Source: CAD feature listing. Evaluate the final solid. Frame: model axes, mm. Face numbers are marked on the shaded views. A direction names the side the tool comes from. Give positions to 0.01 mm unless a question says otherwise; leave off trailing zeros. Write each loop counter-clockwise with the first axis right and the second up, starting at its lowest first coordinate (ties: lowest second). Pieces come first, ordered by that corner, then holes. Notation, with made-up numbers: (32, 3) -> (80, 3) arc R29 ccw to (80, 33) -> close; hole circle Ø11 at (17.5, 64). An arc over 180 degrees is marked (long way). Write item = value, one per line.
from build123d import *

# Parameters (mm, degrees)
SKETCH1_W            = 29.21
SKETCH1_H            = 76.2
BOSS_EXTRUDE1_DEPTH  = 6.858
SKETCH3_R            = 2.032
CUT_EXTRUDE1_DEPTH   = 25.4
SKETCH17_W           = 3.81
SKETCH17_H           = 76.2
BOSS_EXTRUDE13_DEPTH = 67.818
SKETCH18_W           = 3.81
SKETCH18_H           = 20.32
BOSS_EXTRUDE14_DEPTH = 25.4
SKETCH19_W           = 29.21
SKETCH19_H           = 19.948928224
BOSS_EXTRUDE15_DEPTH = 25.4
SKETCH4_R            = 2.032
CUT_EXTRUDE5_DEPTH   = 116.113658891
SKETCH21_R           = 4
SKETCH21_R_2         = 2
CUT_EXTRUDE6_DEPTH   = 3.048
CUT_EXTRUDE7_START   = -3.048
SKETCH22_R           = 4
CUT_EXTRUDE7_DEPTH   = 3.048
SKETCH23_W           = 15.24
SKETCH23_H           = 38.1
CUT_EXTRUDE8_DEPTH   = 109.488248995
SKETCH24_W           = 24.012467883
SKETCH24_H           = 25.448429418
CUT_EXTRUDE9_DEPTH   = 10.16


with BuildPart() as part:
    # Sketch1 → Boss-Extrude1 (new body)
    with BuildSketch(Plane.XY):
        with Locations((19.297661272, -42.679075546)):
            Rectangle(SKETCH1_W, SKETCH1_H)
    extrude(amount=BOSS_EXTRUDE1_DEPTH)

    # Sketch3 → Cut-Extrude1 (cut)
    with BuildSketch(Plane.XY.offset(6.858)):
        with Locations((17.413506863, -42.679058438)):
            Circle(SKETCH3_R)
        with Locations((17.392661272, -29.979075546)):
            Circle(SKETCH3_R)
        with Locations((17.392661272, -17.279075546)):
            Circle(SKETCH3_R)
    extrude(amount=-CUT_EXTRUDE1_DEPTH, mode=Mode.SUBTRACT)

    # Sketch17 → Boss-Extrude13 (add)
    with BuildSketch(Plane(origin=(0, 0, 0), x_dir=(-1, 0, 0), z_dir=(0, 0, -1))):
        with Locations((-31.997661272, -42.679075546)):
            Rectangle(SKETCH17_W, SKETCH17_H)
    extrude(amount=BOSS_EXTRUDE13_DEPTH)

    # Sketch18 → Boss-Extrude14 (add)
    with BuildSketch(Plane.ZY.offset(-30.092661272)):
        with Locations((-65.913, -70.619075546)):
            Rectangle(SKETCH18_W, SKETCH18_H)
    extrude(amount=BOSS_EXTRUDE14_DEPTH)

    # Sketch19 → Boss-Extrude15 (add)
    with BuildSketch(Plane.ZY.offset(-30.092661272)):
        with Locations((-36.703, -70.804611434)):
            Rectangle(SKETCH19_W, SKETCH19_H)
    extrude(amount=BOSS_EXTRUDE15_DEPTH)

    # Sketch4 → Cut-Extrude5 (cut, through all)
    with BuildSketch(Plane.XY.offset(6.858)):
        with Locations((17.413506863, -68.079058438)):
            Circle(SKETCH4_R)
    extrude(amount=-CUT_EXTRUDE5_DEPTH, mode=Mode.SUBTRACT)

    # Sketch21 → Cut-Extrude6 (cut)
    with BuildSketch(Plane(origin=(0, 0, 0), x_dir=(-1, 0, 0), z_dir=(0, 0, -1))):
        with Locations((-17.413506863, -68.079058438)):
            Circle(SKETCH21_R)
        with Locations((-17.413506863, -68.079058438)):
            Circle(SKETCH21_R_2, mode=Mode.SUBTRACT)
    extrude(amount=-CUT_EXTRUDE6_DEPTH, mode=Mode.SUBTRACT)

    # Sketch22 → Cut-Extrude7 (cut)
    with BuildSketch(Plane.XY.offset(6.858).offset(CUT_EXTRUDE7_START)):
        with Locations(Location((17.413506863, -68.079058438, 0), (0, 0, 180))):
            Circle(SKETCH22_R)
    extrude(amount=CUT_EXTRUDE7_DEPTH, mode=Mode.SUBTRACT)

    # Sketch23 → Cut-Extrude8 (cut, through all)
    with BuildSketch(Plane.ZY.offset(-30.092661272)):
        with Locations((-7.62, -61.729075546)):
            Rectangle(SKETCH23_W, SKETCH23_H)
    extrude(amount=-CUT_EXTRUDE8_DEPTH, mode=Mode.SUBTRACT)

    # Sketch24 → Cut-Extrude9 (cut)
    with BuildSketch(Plane.XZ.offset(80.779075546)):
        with Locations((18.088627796, -36.808482529)):
            Rectangle(SKETCH24_W, SKETCH24_H)
    extrude(amount=-CUT_EXTRUDE9_DEPTH, mode=Mode.SUBTRACT)


solid = part.part
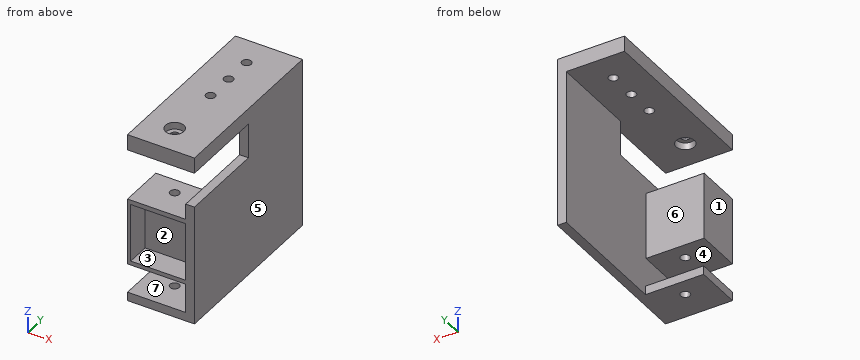
1) Cut plane B-B (x = 24.5). Return the cut outline in (y, z), then the cut area to 3 significant figures.
Computed:
outline = (-80.78, -67.82) -> (-60.46, -67.82) -> (-60.46, -64.01) -> (-80.78, -64.01) -> close; (-80.78, -51.31) -> (-60.83, -51.31) -> (-60.83, -22.1) -> (-80.78, -22.1) -> (-80.78, -24.08) -> (-70.62, -24.08) -> (-70.62, -49.53) -> (-80.78, -49.53) -> close; (-80.78, 0) -> (-4.58, 0) -> (-4.58, 6.86) -> (-80.78, 6.86) -> close
area = 924 mm²
2) Cut plane D-D (z = -48). Return the cut outline in (x, y).
Computed:
outline = (4.69, -80.78) -> (6.08, -80.78) -> (6.08, -70.62) -> (30.09, -70.62) -> (30.09, -80.78) -> (33.9, -80.78) -> (33.9, -4.58) -> (30.09, -4.58) -> (30.09, -60.83) -> (4.69, -60.83) -> close; hole circle Ø4.06 at (17.41, -68.08)
3) Access query for the marked faces 5, 6 and 7. Directions: +Z, -Z, +X, -X, +Y, -Y. A direction counts if a zero-diameter tool reaches every point of the face in a straight line with its end or side. Return the directions, or none.
Computed:
face_5 = +Z, -Z, +X, +Y, -Y
face_6 = -X, +Y
face_7 = -X, +Y, -Y
4) Cut plane C-C (y = -49.5). Return the cut outline in (x, z).
Computed:
outline = (4.69, 0) -> (33.9, 0) -> (33.9, 6.86) -> (4.69, 6.86) -> close; (30.09, -67.82) -> (33.9, -67.82) -> (33.9, -15.24) -> (30.09, -15.24) -> close
5) Cut plane A-A (y = -74). Return the cut outline in (x, z).
Computed:
outline = (4.69, -67.82) -> (33.9, -67.82) -> (33.9, -15.24) -> (30.09, -15.24) -> (30.09, -22.1) -> (4.69, -22.1) -> (4.69, -51.31) -> (30.09, -51.31) -> (30.09, -64.01) -> (4.69, -64.01) -> close; (4.69, 0) -> (33.9, 0) -> (33.9, 6.86) -> (4.69, 6.86) -> close; hole (6.08, -49.53) -> (30.09, -49.53) -> (30.09, -24.08) -> (6.08, -24.08) -> close
6) Contact query for flat-ended pins moving along their axis: pin 1 (14.5 mm diameter, centred on x = 19.5, y = -60, fed in from -Z); pin 2 (4 mm diameter, centred on x = 18, y = -66.5, fed in from +Z); pin 3 (1 mm diameter, centred on x = 27, z = -41.5, fed in from +Y); pin 4 (12 mm diameter, centred on x = 18.5, z = -37, fed in from -Y). Output: stop coordinate, or through.
Computed:
pin_1 = -67.82
pin_2 = 3.81
pin_3 = -60.83
pin_4 = -70.62
7) Material intervals for L1, parallel to Z at x = 13.5, y = -76; L2, parallel to Z at x = 32, y = -50; L3, parallel to X at y = -73, z = -39.5, sorted ascending.
Computed:
L1 = -67.82 to -64.01, -51.31 to -49.53, -24.08 to -22.1, 0 to 6.86
L2 = -67.82 to -15.24, 0 to 6.86
L3 = 4.69 to 6.08, 30.09 to 33.9
8) Draft query along X for the marked faces 1, 2, 3 and 4. Return one class per face: pulls with the +X half, pulls with the -X half, needs draft (parallel to the pull), parting line crosses it, or undercut.
Computed:
face_1 = pulls with the -X half
face_2 = undercut
face_3 = undercut
face_4 = needs draft
